```python
from build123d import *

# Parameters (mm, degrees)
SKETCH1_W           = 44.45
SKETCH1_H           = 44.45
SKETCH1_W_2         = 38.1
SKETCH1_H_2         = 38.1
BOSS_EXTRUDE1_DEPTH = 628.65
CUT_EXTRUDE1_REACH  = 46.45


with BuildPart() as part:
    # Sketch1 → Boss-Extrude1 (new body, symmetric)
    with BuildSketch(Plane(origin=(0, 0, 0), x_dir=(0, 0, -1), z_dir=(1, 0, 0))):
        with Locations((22.225, 22.225)):
            Rectangle(SKETCH1_W, SKETCH1_H)
        with Locations((22.225, 22.225)):
            Rectangle(SKETCH1_W_2, SKETCH1_H_2, mode=Mode.SUBTRACT)
    extrude(amount=BOSS_EXTRUDE1_DEPTH, both=True)

    # Sketch2 → Cut-Extrude1 (cut, up to next)
    with BuildSketch(Plane.XY, mode=Mode.PRIVATE) as cut_extrude1_sk1:
        with BuildLine():
            Line((-196.723, 12.827), (-184.277, 12.827))
            ThreePointArc((-184.277, 12.827), (-180.975, 9.525), (-184.277, 6.223))
            Line((-184.277, 6.223), (-196.723, 6.223))
            ThreePointArc((-196.723, 6.223), (-200.025, 9.525), (-196.723, 12.827))
        make_face()
    cut_extrude1_tool1 = extrude(cut_extrude1_sk1.sketch, amount=-CUT_EXTRUDE1_REACH, mode=Mode.PRIVATE) & part.part
    add(cut_extrude1_tool1.solids().sort_by_distance((-190.5, 9.525, 0))[0], mode=Mode.SUBTRACT)
    # Sketch2 → Cut-Extrude1 (cut, up to next)
    with BuildSketch(Plane.XY, mode=Mode.PRIVATE) as cut_extrude1_sk2:
        with BuildLine():
            Line((-69.723, 12.827), (-57.277, 12.827))
            ThreePointArc((-57.277, 12.827), (-53.975, 9.525), (-57.277, 6.223))
            Line((-57.277, 6.223), (-69.723, 6.223))
            ThreePointArc((-69.723, 6.223), (-73.025, 9.525), (-69.723, 12.827))
        make_face()
    cut_extrude1_tool2 = extrude(cut_extrude1_sk2.sketch, amount=-CUT_EXTRUDE1_REACH, mode=Mode.PRIVATE) & part.part
    add(cut_extrude1_tool2.solids().sort_by_distance((-63.5, 9.525, 0))[0], mode=Mode.SUBTRACT)


solid = part.part
```
Can you work these out from the model? Positions are in its coordinate system, mm. A direction names the side the tool comes from. Round coordinates to 2 decimals unless told otherwise and drop trailing zeros. Loops run counter-clockwise (first coordinate to the right, second up) from the corner with the lowest first, then second, coordinate; pieces in that order, holes last. Notation, with made-up numbers: M 37,32.5 L 96,32.5 A17 cw 96,39.5 Z; hole C -26,30.5 d11. An arc over 180 degrees is marked long. Write item = value, one per line. Start each with the question number.
(1) Suppose I cut it at B-B on x = -233. Write out the boundary of the cut face in (y, z) (3 decimals).
(2) I'm going to push a flat-ended pin straight in: P1, Ø19, axis at x = -116.5, y = 29, coming from the +Z side. Where does the tip first touch, or does it pass through?
(3) If we mould it in two halves opening along Y, with no side actions, what happens to faces 1 (the face through (9, 22, -3.175)), 2 (the face through (9, 22, -44.45)), 3 (the face through (9, 0, -22)), 4 (the face through (9, 41.275, -22))? For each: released by +Y, released by -Y, zero draft, split by the parting line, or undercut.
(4) I need wall thicknesses on line 1 along Y through (x, z) = (-50, -17) (3 decimals); line 2 along Z through (x, y) = (286, 32) (3 decimals). Which ranges of each line are inside material? Lowest first, please.
(5) Suppose I cut it at A-A on y = 24. Write out the boundary of the cut face in (x, z) (3 decimals), plus the area to 3 significant figures.
(6) Suppose I cut it at C-C on z = -26. Write out the boundary of the cut face in (x, y) (3 decimals), plus the area to 3 significant figures.
(7) Which directions (+Z, -Z, +X, -X, +Y, -Y) give clear straight access to the entire face, cutting with the end or side of a thin tool? Please do faces 5 (the face through (9, 22, -41.275)), 6 (the face through (9, 44.45, -22)).
Answer block:
q1.outline = M 0,-44.45 L 44.45,-44.45 L 44.45,0 L 0,0 Z; hole M 3.175,-41.275 L 41.275,-41.275 L 41.275,-3.175 L 3.175,-3.175 Z
q2.P1 = 0
q3.face_1 = undercut
q3.face_2 = zero draft
q3.face_3 = released by -Y
q3.face_4 = undercut
q4.line_1 = 0 to 3.175, 41.275 to 44.45
q4.line_2 = -44.45 to -41.275, -3.175 to 0
q5.outline = M -628.65,-44.45 L 628.65,-44.45 L 628.65,-41.275 L -628.65,-41.275 Z; M -628.65,-3.175 L 628.65,-3.175 L 628.65,0 L -628.65,0 Z
q5.area = 7,980 mm²
q6.outline = M -628.65,0 L 628.65,0 L 628.65,3.175 L -628.65,3.175 Z; M -628.65,41.275 L 628.65,41.275 L 628.65,44.45 L -628.65,44.45 Z
q6.area = 7,980 mm²
q7.face_5 = +X, -X
q7.face_6 = +Z, -Z, +X, -X, +Y
